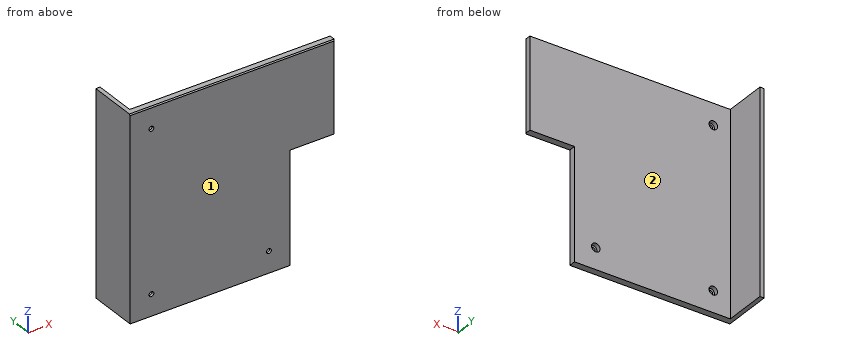
from build123d import *

# Parameters (mm, degrees)
SKETCH1_W                      = 192.4
SKETCH1_H                      = 190
BOSS_EXTRUDE1_DEPTH            = 6.35
BOSS_EXTRUDE2_DEPTH            = 40
CUT_EXTRUDE1_REACH             = 8.35
SKETCH4_W                      = 42
SKETCH4_H                      = 104.6
CBORE_FOR_M4_SHCS1_D           = 4.5
CBORE_FOR_M4_SHCS1_DEPTH       = 6.35
CBORE_FOR_M4_SHCS1_CBORE_D     = 8
CBORE_FOR_M4_SHCS1_CBORE_DEPTH = 4
CHAMFER1_SIZE                  = 1


with BuildPart() as part:
    # Sketch1 → Boss-Extrude1 (new body)
    with BuildSketch(Plane(origin=(0, 0, 0), x_dir=(1, 0, 0), z_dir=(0, 1, 0))):
        Rectangle(SKETCH1_W, SKETCH1_H)
    extrude(amount=BOSS_EXTRUDE1_DEPTH)

    # Sketch2 → Boss-Extrude2 (add)
    with BuildSketch(Plane(origin=(0, 6.35, 0), x_dir=(1, 0, 0), z_dir=(0, 1, 0))):
        Polygon((-92.2, 91), (-92.2, -91), (-92.2, -95), (-96.2, -95), (-96.2, 95), (-92.2, 95), align=None)
    extrude(amount=BOSS_EXTRUDE2_DEPTH)

    # Sketch4 → Cut-Extrude1 (cut, up to next)
    with BuildSketch(Plane(origin=(0, 6.35, 0), x_dir=(1, 0, 0), z_dir=(0, 1, 0)), mode=Mode.PRIVATE) as cut_extrude1_sk1:
        with Locations((75.2, 42.7)):
            Rectangle(SKETCH4_W, SKETCH4_H)
    cut_extrude1_tool1 = extrude(cut_extrude1_sk1.sketch, amount=-CUT_EXTRUDE1_REACH, mode=Mode.PRIVATE) & part.part
    add(cut_extrude1_tool1.solids().sort_by_distance((75.2, 6.35, -42.7))[0], mode=Mode.SUBTRACT)

    # CBORE for M4 SHCS1
    with Locations(Plane(origin=(0, 6.35, 0), x_dir=(1, 0, 0), z_dir=(0, 1, 0))):
        with Locations((34.2, 75), (-76.2, 75), (-76.2, -75)):
            CounterBoreHole(CBORE_FOR_M4_SHCS1_D / 2, CBORE_FOR_M4_SHCS1_CBORE_D / 2, CBORE_FOR_M4_SHCS1_CBORE_DEPTH, depth=CBORE_FOR_M4_SHCS1_DEPTH)

    # Chamfer1
    chamfer1_edges = [part.edges().sort_by_distance(p)[0] for p in [
        (0, 0, 95),
        (96.2, 0, 52.3),
    ]]
    chamfer(chamfer1_edges, length=CHAMFER1_SIZE)


solid = part.part
Check sheet for the modelled part. Datum: model origin and axes. Units: mm. Face numbers are marked on the shaded views. A direction names the side the tool comes from. Round coordinates to 2 decimals unless told otherwise and drop trailing zeros. Order: outer loops, then holes, each group sorted by start corner. A loop starts at its lowest first (then second) coordinate and runs counter-clockwise, first axis right, second up.
Q1. Depth check by flat-ended pin: P1, Ø12, axis at x = -20.5, z = 44.5, coming from the +Y side; P2, Ø10.5, axis at x = -76.2, z = -75, coming from the -Y side; P3, Ø8, axis at y = 23.5, z = 74.5, coming from the +X side; P4, Ø6, axis at x = 34.2, z = -75, coming from the +Y side. Enter the tip coordinate at first touch or a pass-through.
Filled sheet:
P1: stops at y = 6.35
P2: stops at y = 0
P3: stops at x = -92.2
P4: stops at y = 2.35
Q2. Cross-section at A-A, the plane z = 75. Enter the section's corners in (x, y).
Filled sheet:
outline: (-96.2, 0) - (-78.45, 0) - (-78.45, 2.35) - (-80.2, 2.35) - (-80.2, 6.35) - (-92.2, 6.35) - (-92.2, 46.35) - (-96.2, 46.35) - close; (-73.95, 0) - (95.2, 0) - (96.2, 1) - (96.2, 6.35) - (-72.2, 6.35) - (-72.2, 2.35) - (-73.95, 2.35) - close
Q3. Cross-section at D-D, the plane z = -75. Enter the section's corners in (x, y), plus the area to 3 significant figures.
Filled sheet:
outline: (-96.2, 0) - (-78.45, 0) - (-78.45, 2.35) - (-80.2, 2.35) - (-80.2, 6.35) - (-92.2, 6.35) - (-92.2, 46.35) - (-96.2, 46.35) - close; (-73.95, 0) - (31.95, 0) - (31.95, 2.35) - (30.2, 2.35) - (30.2, 6.35) - (-72.2, 6.35) - (-72.2, 2.35) - (-73.95, 2.35) - close; (36.45, 0) - (54.2, 0) - (54.2, 6.35) - (38.2, 6.35) - (38.2, 2.35) - (36.45, 2.35) - close
area: 1,030 mm2
Q4. Cross-section at B-B, the plane x = 34.2. Enter the section's corners in (y, z).
Filled sheet:
outline: (0, -95) - (6.35, -95) - (6.35, -79) - (2.35, -79) - (2.35, -77.25) - (0, -77.25) - close; (0, -72.75) - (2.35, -72.75) - (2.35, -71) - (6.35, -71) - (6.35, 95) - (1, 95) - (0, 94) - close
Q5. Set-up check for the marked faces 1 and 2: record each of +Z, -Z, +X, -X, +Y, -Y from which the full face is reachable in a straight line by a thin tool's end or side.
Filled sheet:
face 1: +Z, -Z, +X, -X, -Y
face 2: +Z, -Z, +X, +Y
Q6. Cross-section at C-C, the plane x = -76.2. Enter the section's corners in (y, z), plus the area to 3 significant figures.
Filled sheet:
outline: (0, -95) - (6.35, -95) - (6.35, -79) - (2.35, -79) - (2.35, -77.25) - (0, -77.25) - close; (0, -72.75) - (2.35, -72.75) - (2.35, -71) - (6.35, -71) - (6.35, 71) - (2.35, 71) - (2.35, 72.75) - (0, 72.75) - close; (0, 77.25) - (2.35, 77.25) - (2.35, 79) - (6.35, 79) - (6.35, 95) - (1, 95) - (0, 94) - close
area: 1,120 mm2
Q7. Scan lines: L1, parallel to X at y = 0.6, z = -75; L2, parallel to X at y = 1.35, z = 75; L3, parallel to Y at x = 87, z = 70. Record each from-to range of solid material in increasing order.
Filled sheet:
L1: x = -96.2 to -78.45, -73.95 to 31.95, 36.45 to 54.2
L2: x = -96.2 to -78.45, -73.95 to 96.2
L3: y = 0 to 6.35
